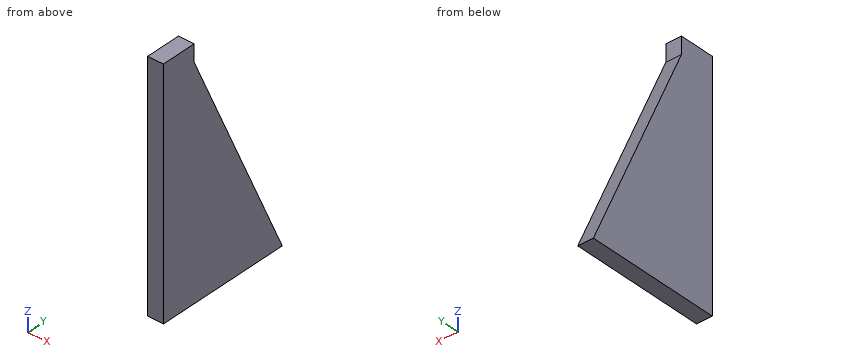
```python
from build123d import *

# Parameters (mm, degrees)
F1_DEPTH = 4.7625


# Not quite as in the source:
# - a length typed as a fraction of an inch, garbled in the dataset ("3 / 203.2 mm" for 3/8 in), is restored


with BuildPart() as f1:
    # F0 (on Right) → F1 (new body, symmetric)
    with BuildSketch(Plane.YZ):
        Polygon((21.5, 62.8277051401), (0, 62.8277051401), (0, -82.1722948599), (82.89, -82.1722948599), (21.5, 52.4577051401), align=None)
    extrude(amount=F1_DEPTH, both=True)


solid = f1.part
```
Geometry check sheet. Reference: the model listing, model coordinates, mm. Give positions to 0.01 mm unless a question says otherwise; leave off trailing zeros. Write each loop counter-clockwise with the first axis right and the second up, starting at its lowest first coordinate (ties: lowest second). Pieces come first, ordered by that corner, then holes.
1) Gauge pin test, flat ends, axial feed: pin 1 (2 mm diameter, centred on x = -2, y = 70.5, fed in from +Z); pin 2 (3 mm diameter, centred on x = 1, y = 70, fed in from +Z); pin 3 (3 mm diameter, centred on x = -2.5, z = 58, fed in from +Y). Record the tip position at first contact, or that the pin passes through.
2) Section check B-B, the plane z = 3. Record the boundary of the cut face in (x, y), and give its area (3 significant figures).
3) Section check A-A, the plane x = 2.25. Record the boundary of the cut face in (y, z), and give its area (3 significant figures).
4) Material ranges on L1, parallel to Z at x = 2.25, y = 70; L2, parallel to Y at x = -0.5, z = 20; L3, parallel to Y at x = 0.5, z = -64, recorded low to high.
5) Section check C-C, the plane y = 23.5. Record the boundary of the cut face in (x, z).
Computed:
1. pin 1: stops at z = -52.81
1. pin 2: stops at z = -50.61
1. pin 3: stops at y = 21.5
2. outline: (-4.76, 0) - (4.76, 0) - (4.76, 44.05) - (-4.76, 44.05) - close
2. area: 420 mm2
3. outline: (0, -82.17) - (82.89, -82.17) - (21.5, 52.46) - (21.5, 62.83) - (0, 62.83) - close
3. area: 7,250 mm2
4. L1: z = -82.17 to -53.9
4. L2: y = 0 to 36.3
4. L3: y = 0 to 74.6
5. outline: (-4.76, -82.17) - (4.76, -82.17) - (4.76, 48.07) - (-4.76, 48.07) - close
